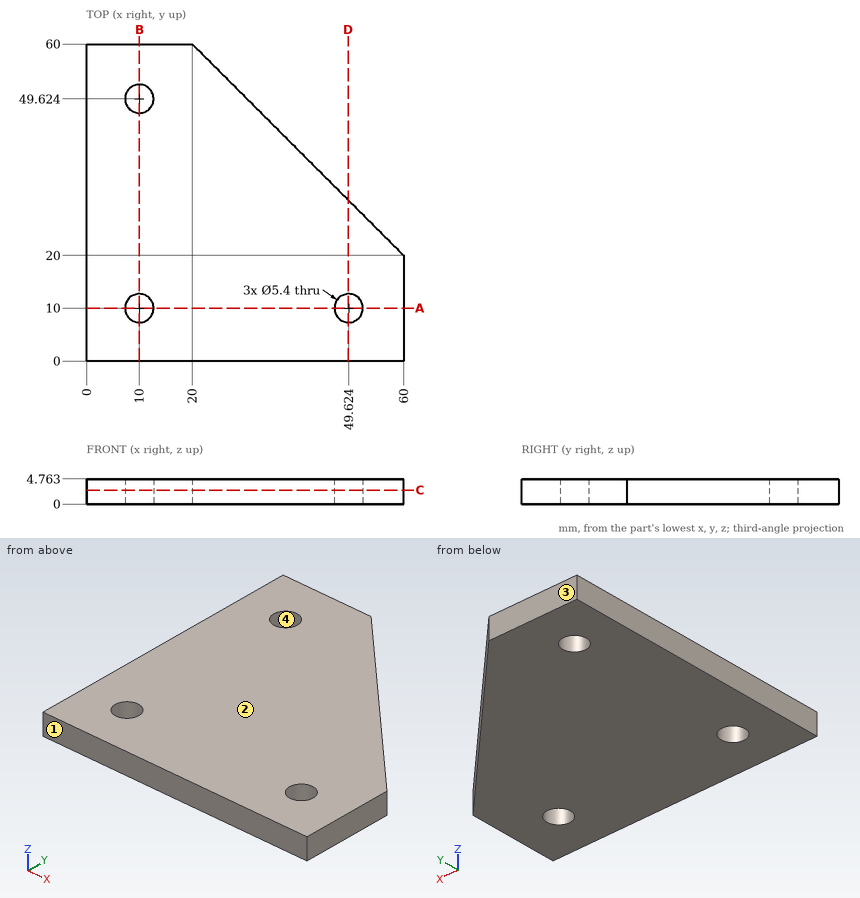
The figure shows three views and two pictorial views of one solid part (mm, origin at its lowest corner). Answer the questions. Coordinates: 2 decimals unless noted, no trailing zeros. Loops run counter-clockwise (first coordinate to the right, second up) from the corner with the lowest first, then second, coordinate; pieces in that order, holes last. Notation, with made-up numbers: (-25, 83.5) -> (13, 83.5) arc R23 ccw to (13, 112.5) -> close; hole circle Ø9 at (34.25, -20). An arc over 180 degrees is marked (long way). Use one line per item in the form item = value. Start each with the question number.
Item 1: The part is cut by section C-C on z = 2.65. Determine the outline of the cut face in (x, y) (1 decimal).
Item 2: Consider L1, parallel to Y at x = 10, z = 1.6 (1 decimal); L2, parallel to Y at x = 51, z = 4.3 (1 decimal). Determine where each line is inside the solid, lowest interval first. Write a range as [from, to].
Item 3: Flat-ended cylindrical pins translate along their axes: pin 1 Ø4.5 at (x, y) = (10, 49.624) entering from -Z; pin 2 Ø2 at (y, z) = (31, 0.5) entering from +X. Find the tip coordinate at first contact, or state that the pin passes through.
Item 4: The part is cut by section D-D on x = 49.5. Determine the outline of the cut face in (y, z).
Item 5: The part is cut by section A-A on y = 10. Determine the outline of the cut face in (x, z) (1 decimal), then the cut area to 3 significant figures.
Item 6: The mould has two halves that part along Y. Classify the marked faces 1, 2, 3 and 4: released by +Y, released by -Y, zero draft, split by the parting line, or undercut.
Answer key:
q1.outline = (0, 0) -> (60, 0) -> (60, 20) -> (20, 60) -> (0, 60) -> close; hole circle Ø5.4 at (10, 10); hole circle Ø5.4 at (10, 49.6); hole circle Ø5.4 at (49.6, 10)
q2.L1 = [0, 7.3], [12.7, 46.9], [52.3, 60]
q2.L2 = [0, 7.7], [12.3, 29]
q3.pin_1 = through
q3.pin_2 = 50
q4.outline = (0, 0) -> (7.3, 0) -> (7.3, 4.76) -> (0, 4.76) -> close; (12.7, 0) -> (30.5, 0) -> (30.5, 4.76) -> (12.7, 4.76) -> close
q5.outline = (0, 0) -> (7.3, 0) -> (7.3, 4.8) -> (0, 4.8) -> close; (12.7, 0) -> (46.9, 0) -> (46.9, 4.8) -> (12.7, 4.8) -> close; (52.3, 0) -> (60, 0) -> (60, 4.8) -> (52.3, 4.8) -> close
q5.area = 234 mm2
q6.face_1 = released by -Y
q6.face_2 = zero draft
q6.face_3 = released by +Y
q6.face_4 = undercut
